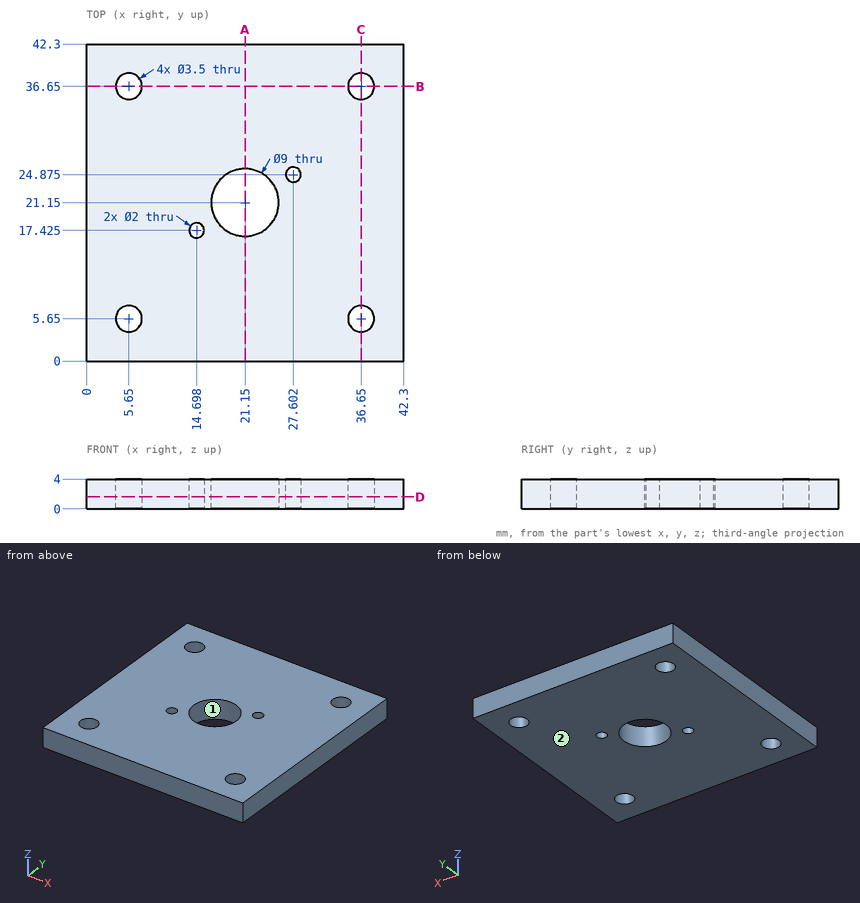
Design review of the part shown in the three views and the two pictorial views. Dimensions are in mm from the part's minimum x, y and z. Round coordinates to 2 decimals unless told otherwise and drop trailing zeros. Loops run counter-clockwise (first coordinate to the right, second up) from the corner with the lowest first, then second, coordinate; pieces in that order, holes last. Notation, with made-up numbers: M 66,76.5 L 84,76.5 A22 ccw 84,90.5 Z; hole C 89,-12.5 d9. An arc over 180 degrees is marked long. Write item = value, one per line.
Item 1: Insertion check: P1, Ø3, axis at x = 36.65, y = 36.65, coming from the -Z side. The pin has a flat end and moves straight along its axis. Give the tip position at first contact, or say it passes through.
Return value:
P1 = through
Item 2: Take a section at D-D on z = 1.6. Write out the cut boundary in (x, y) (3 decimals).
Return value:
outline = M 0,0 L 42.3,0 L 42.3,42.3 L 0,42.3 Z; hole C 5.65,5.65 d3.5; hole C 5.65,36.65 d3.5; hole C 14.698,17.425 d2; hole C 21.15,21.15 d9; hole C 27.602,24.875 d2; hole C 36.65,5.65 d3.5; hole C 36.65,36.65 d3.5
Item 3: Take a section at B-B on y = 36.65. Write out the cut boundary in (x, z), then the cut area to 3 significant figures.
Return value:
outline = M 0,0 L 3.9,0 L 3.9,4 L 0,4 Z; M 7.4,0 L 34.9,0 L 34.9,4 L 7.4,4 Z; M 38.4,0 L 42.3,0 L 42.3,4 L 38.4,4 Z
area = 141 mm2
Item 4: Take a section at A-A on x = 21.15. Write out the cut boundary in (y, z), then the cut area to 3 significant figures.
Return value:
outline = M 0,0 L 16.65,0 L 16.65,4 L 0,4 Z; M 25.65,0 L 42.3,0 L 42.3,4 L 25.65,4 Z
area = 133 mm2
Item 5: For line 1 (Y direction, x = 5.65, z = 1.5); line 2 (X direction, y = 37.5, z = 1.25); line 3 (X direction, y = 18, z = 3.85), list the stretches that pass through material, from the lowest coordinate up. Write a range as [from, to].
Return value:
line_1 = [0, 3.9], [7.4, 34.9], [38.4, 42.3]
line_2 = [0, 4.12], [7.18, 35.12], [38.18, 42.3]
line_3 = [0, 13.88], [15.52, 17.94], [24.36, 42.3]
Item 6: The part is to be moulded in two halves that separate along X. For the marked faces 1 and 2, say which applies: released by +X, released by -X, zero draft, split by the parting line, or undercut.
Return value:
face_1 = undercut
face_2 = zero draft
